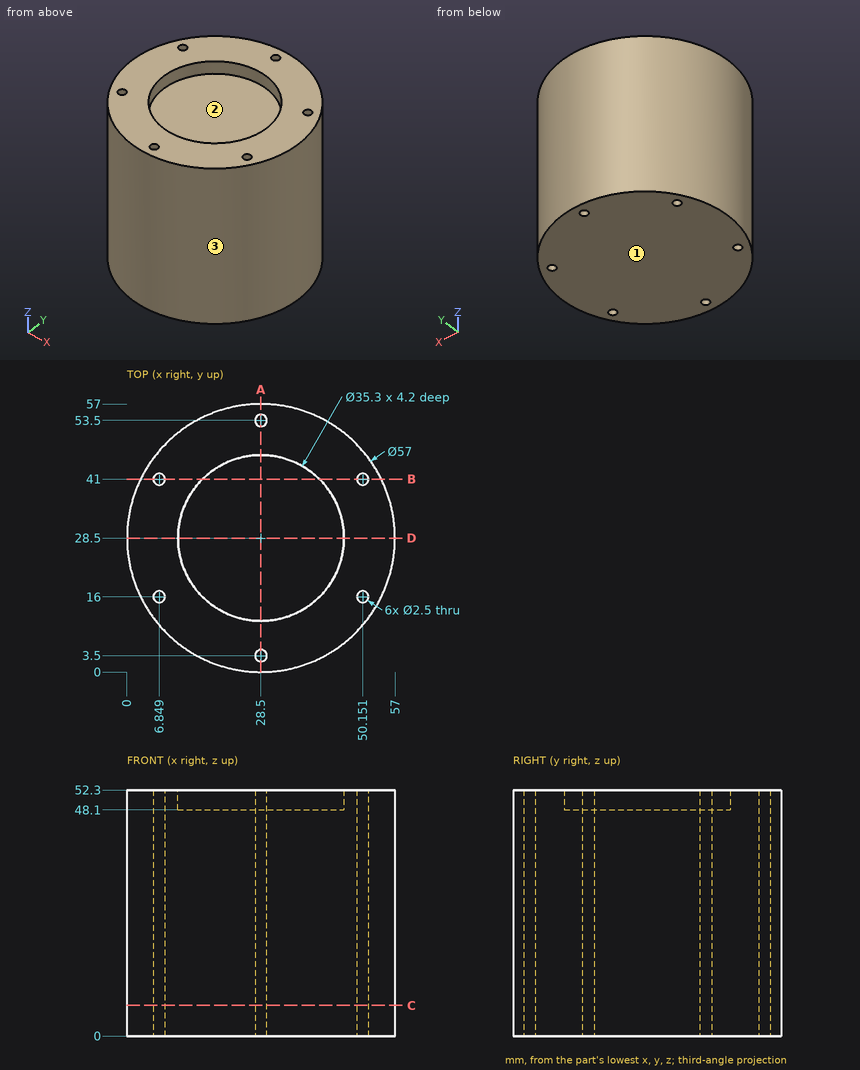
Input: dimensioned drawing with shaded views. Units: mm. Origin: part minimum x, y, z. Round coordinates to 2 decimals unless told otherwise and drop trailing zeros. Order: outer loops, then holes, each group sorted by start corner. A loop starts at its lowest first (then second) coordinate and runs counter-clockwise, first axis right, second up. Notation, with made-up numbers: (84.5, -3) - (115.5, -3) arc R18 cw to (115.5, 30) - close; hole circle Ø10 at (6, 79.5). An arc over 180 degrees is marked (long way). Write item = value, one per line. Start each with the question number.
Q1. Cut plane C-C on z = 6.5. Return the cut outline in (x, y).
Q2. Cut plane B-B on y = 41. Return the cut outline in (x, z).
Q3. Cut plane A-A on x = 28.5. Return the cut outline in (y, z).
Q4. Ray query, line 1 (X direction, y = 15.5, z = 18) (1 decimal); line 2 (Y direction, x = 7.5, z = 22) (1 decimal); line 3 (X direction, y = 41, z = 24). Return the intervals inside material, ascending. Write a range as from..to.
Q5. Cut plane D-D on y = 28.5. Return the cut outline in (x, z), and give its area (3 significant figures).
Q6. Pin query (flat end, axial travel): pin 1 (5 mm diameter, centred on y = 33, z = 44.5, fed in from +X); pin 2 (12 mm diameter, centred on x = 46, z = 25, fed in from -Y); pin 3 (6 mm diameter, centred on y = 34, z = 37.5, fed in from -X). Return the tip coordinate at first contact, or that it passes through.
Q7. Pull-direction query (Y, two-part tool) for the marked faces 1, 2 and 3; classes: +Y half, -Y half, draft (parallel to the pull), parting line (faces both ways), or undercut.
Outcome:
q1.outline = circle Ø57 at (28.5, 28.5); hole circle Ø2.5 at (6.85, 16); hole circle Ø2.5 at (6.85, 41); hole circle Ø2.5 at (28.5, 3.5); hole circle Ø2.5 at (28.5, 53.5); hole circle Ø2.5 at (50.15, 16); hole circle Ø2.5 at (50.15, 41)
q2.outline = (2.89, 0) - (5.6, 0) - (5.6, 52.3) - (2.89, 52.3) - close; (8.1, 0) - (48.9, 0) - (48.9, 52.3) - (40.96, 52.3) - (40.96, 48.1) - (16.04, 48.1) - (16.04, 52.3) - (8.1, 52.3) - close; (51.4, 0) - (54.11, 0) - (54.11, 52.3) - (51.4, 52.3) - close
q3.outline = (0, 0) - (2.25, 0) - (2.25, 52.3) - (0, 52.3) - close; (4.75, 0) - (52.25, 0) - (52.25, 52.3) - (46.15, 52.3) - (46.15, 48.1) - (10.85, 48.1) - (10.85, 52.3) - (4.75, 52.3) - close; (54.75, 0) - (57, 0) - (57, 52.3) - (54.75, 52.3) - close
q4.line_1 = 3.1..5.7, 8..49, 51.3..53.9
q4.line_2 = 9.2..14.9, 17.1..39.9, 42.1..47.8
q4.line_3 = 2.89..5.6, 8.1..48.9, 51.4..54.11
q5.outline = (0, 0) - (57, 0) - (57, 52.3) - (46.15, 52.3) - (46.15, 48.1) - (10.85, 48.1) - (10.85, 52.3) - (0, 52.3) - close
q5.area = 2,830 mm^2
q6.pin_1 = 56.93
q6.pin_2 = 2.42
q6.pin_3 = 0.11
q7.face_1 = draft
q7.face_2 = undercut
q7.face_3 = parting line
